Read the model definition and answer for the solid it produces. Units are mm, in the model's axes. Coordinates: 2 decimals unless noted, no trailing zeros. Loops run counter-clockwise (first coordinate to the right, second up) from the corner with the lowest first, then second, coordinate; pieces in that order, holes last. Notation, with made-up numbers: M 70,84 L 92,84 A21 cw 92,101 Z; hole C 7,16.25 d6. An arc over 180 degrees is marked long. Use one line per item in the form item = value. Start each with the question number.
1. The part is cut by section A-A (y = 28). Give the vertices of the cut face in (x, z), plus the area to 3 significant figures.
2. The part is cut by section B-B (z = 421). Give the vertices of the cut face in (x, y), plus the area to 3 significant figures.
3. Find the intervals of material crossed by probe 1 along X at (y, z) = (107, 184); probe 2 along Z at (x, y) = (285, 86), in increasing order. Write a range as [from, to].
4. Flat-ended cylindrical pins translate along their axes: pin 1 (12 mm diameter, centred on y = 191, z = 435.5, fed in from +X); pin 2 (7.5 mm diameter, centred on y = 69, z = 814, fed in from +X); pin 3 (22.5 mm diameter, centred on x = 333.5, z = 705.5, fed in from -Y). Find the tip coordinate at first contact, or state that the pin passes through.
from build123d import *

# Parameters (mm, degrees)
F0_W        = 600
F0_H        = 500
F1_DEPTH    = 800
F2_W        = 500
F2_H        = 80
F3_DEPTH    = 25
F5_DEPTH    = 50
F6_T1_DEPTH = 120
F6_T4_ANGLE = 180
F6_T6_ANGLE = 180
F7_W        = 40
F7_H        = 110
F8_DEPTH    = 25
F9_R        = 4.99999
F10_W       = 630
F10_H       = 500
F11_DEPTH   = 25


# Not quite as in the source:
# - a fillet or chamfer that OpenCascade refuses, or shapes differently, is made with other operations: its cross-section is extruded or revolved along the edge and cut away or added
# - a fillet or chamfer is up to 0.001 mm smaller than in the source, because OpenCascade refuses the exact size


with BuildPart() as f1:
    # F0 (on Top) → F1 (new body)
    with BuildSketch(Plane.XY):
        Rectangle(F0_W, F0_H)
    extrude(amount=F1_DEPTH)

    # F2 (on face) → F3 (cut)
    with BuildSketch(Plane.YZ.offset(300)):
        with Locations((0, 40)):
            Rectangle(F2_W, F2_H)
    extrude(amount=-F3_DEPTH, mode=Mode.SUBTRACT)

    # F4 (on face) → F5 (join)
    with BuildSketch(Plane.YZ.offset(300)):
        with BuildLine():
            ThreePointArc((-220, 750), (-223.5355339059, 748.5355339059), (-225, 745))
            Line((-225, 745), (-225, 625))
            ThreePointArc((-225, 625), (-223.5355339059, 621.4644660941), (-220, 620))
            ThreePointArc((-220, 620), (-216.4644660941, 621.4644660941), (-215, 625))
            Line((-215, 625), (-215, 745))
            ThreePointArc((-215, 745), (-216.4644660941, 748.5355339059), (-220, 750))
        make_face()
    extrude(amount=F5_DEPTH)

    # F6: fillet of radius 5 on 4 edges, made by hand

    # F6_s2 → F6_t1 (cut)
    with BuildSketch(Plane.XY.offset(625)):
        with BuildLine():
            ThreePointArc((345, -225), (348.5355339059, -223.5355339059), (350, -220))
            Line((350, -220), (350.1, -220))
            Line((350.1, -220), (350.1, -225.1))
            Line((350.1, -225.1), (345, -225.1))
            Line((345, -225.1), (345, -225))
        make_face()
        with BuildLine():
            ThreePointArc((345, -215), (348.5355339059, -216.4644660941), (350, -220))
            Line((350, -220), (350.1, -220))
            Line((350.1, -220), (350.1, -214.9))
            Line((350.1, -214.9), (345, -214.9))
            Line((345, -214.9), (345, -215))
        make_face()
    extrude(amount=F6_T1_DEPTH, mode=Mode.SUBTRACT)

    # F6_s3 → F6_t4 (revolve, cut)
    with BuildSketch(Plane.XY.offset(745)):
        with BuildLine():
            ThreePointArc((345, -225), (348.5355339059, -223.5355339059), (350, -220))
            Line((350, -220), (350.1, -220))
            Line((350.1, -220), (350.1, -225.1))
            Line((350.1, -225.1), (345, -225.1))
            Line((345, -225.1), (345, -225))
        make_face()
    revolve(axis=Axis((350, -220, 745), (-1, 0, 0)), revolution_arc=F6_T4_ANGLE, mode=Mode.SUBTRACT)

    # F6_s5 → F6_t6 (revolve, cut)
    with BuildSketch(Plane.XY.offset(625)):
        with BuildLine():
            ThreePointArc((345, -215), (348.5355339059, -216.4644660941), (350, -220))
            Line((350, -220), (350.1, -220))
            Line((350.1, -220), (350.1, -214.9))
            Line((350.1, -214.9), (345, -214.9))
            Line((345, -214.9), (345, -215))
        make_face()
    revolve(axis=Axis((350, -220, 625), (-1, 0, 0)), revolution_arc=F6_T6_ANGLE, mode=Mode.SUBTRACT)

    # F7 (on face) → F8 (cut)
    with BuildSketch(Plane(origin=(0, -215, 0), x_dir=(-1, 0, 0), z_dir=(0, 1, 0))):
        with Locations((-320, 685)):
            Rectangle(F7_W, F7_H)
    extrude(amount=-F8_DEPTH, mode=Mode.SUBTRACT)

    # F9 (radius 5 in the source; OpenCascade refuses exactly that, so slightly less here)
    f9_edges = [f1.edges().sort_by_distance(p)[0] for p in [
        (320, -215, 740),
        (340, -215, 685),
        (320, -215, 630),
        (320, -225, 740),
        (340, -225, 685),
        (320, -225, 630),
    ]]
    fillet(f9_edges, radius=F9_R)

    # F10 (on face) → F11 (join)
    with BuildSketch(Plane.XY.offset(800)):
        with Locations((15, 0)):
            Rectangle(F10_W, F10_H)
    extrude(amount=F11_DEPTH)


solid = f1.part
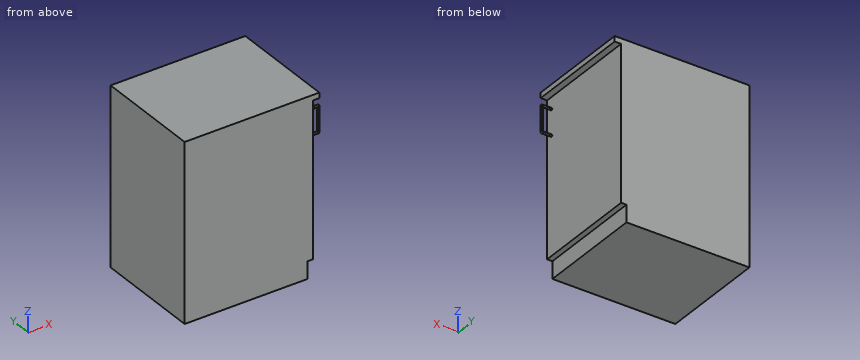
Computed values:
q1.outline = M -300,0 L 275,0 L 275,80 L 300,80 L 300,800 L 330,800 L 330,825 L -300,825 Z
q1.area = 494,000 mm²
q2.outline = M -300,-250 L 300,-250 L 300,250 L -300,250 Z
q2.area = 300,000 mm²
q3.probe_1 = [-300, 300]
q3.probe_2 = [80, 825]
q4.pin_1 = 300
q4.pin_2 = 330
q4.pin_3 = -224.99
